```python
from build123d import *

# Parameters (mm, degrees)
PAD001_DEPTH      = 3.3
SKETCH002_W       = 1.5
SKETCH002_H       = 2.9
POCKET_DEPTH      = 5
PAD002_DEPTH      = 0.1
PAD002_DEPTH_BACK = 1


with BuildPart() as part:
    # Sketch001 → Pad001 (new body)
    with BuildSketch(Plane.XY.offset(0.01)):
        Polygon((-7.95, 11), (7.95, 11), (7.95, 0), (-6.95, 0), (-7.95, 1), align=None)
    extrude(amount=PAD001_DEPTH)

    # Sketch002 → Pocket (cut)
    with BuildSketch(Plane.XY.offset(3.31)):
        with Locations((-7.2, 5.5)):
            Rectangle(SKETCH002_W, SKETCH002_H)
        with Locations((7.2, 5.5)):
            Rectangle(SKETCH002_W, SKETCH002_H)
    extrude(amount=-POCKET_DEPTH, mode=Mode.SUBTRACT)

    # Sketch003 → Pad002 (new body, two sides)
    with BuildSketch(Plane(origin=(0, 0, 0.01), x_dir=(1, 0, 0), z_dir=(0, 0, -1))) as pad002_sk:
        Polygon((-7.95, -6.95), (-7.95, -4.05), (-4.8, -4.05), (-4.8, -2.5), (4.8, -2.5), (4.8, -4.05), (7.95, -4.05), (7.95, -6.95), (4.8, -6.95), (4.8, -8.5), (-4.8, -8.5), (-4.8, -6.95), align=None)
    extrude(amount=PAD002_DEPTH)
    extrude(pad002_sk.sketch, amount=-PAD002_DEPTH_BACK)


solid = part.part
```
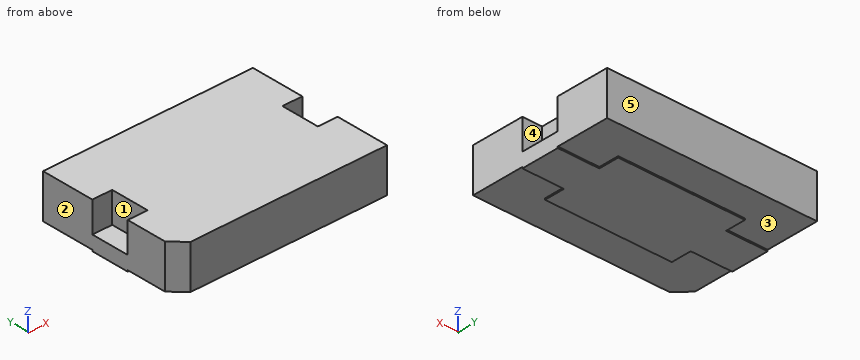
Can you work these out from the model? Positions are in its coordinate system, mm. Face numbers are marked on the shaded views. A direction names the side the tool comes from. Coordinates: 2 decimals unless noted, no trailing zeros. Order: outer loops, then holes, each group sorted by start corner. A loop starts at its lowest first (then second) coordinate and runs counter-clockwise, first axis right, second up. Notation, with made-up numbers: (47.5, 38) - (76.5, 38) arc R29 ccw to (76.5, 77) - close; hole circle Ø8 at (83, 12.5). An arc over 180 degrees is marked (long way). Answer in a Markdown table with one row per item.
1. Suppose I cut it at D-D (y = 1.25). Please give me the cut outline in (x, z), and give its area (3 significant figures).
Reply:
| item | result |
|---|---|
| outline | (-7.95, 0.01) - (7.95, 0.01) - (7.95, 3.31) - (-7.95, 3.31) - close |
| area | 52.5 mm^2 |
2. For the marked faces 1 and 2, which set-ups out of +Z, -Z, +X, -X, +Y, -Y let a thin tool reach every point of the face, with its end or its side?
Reply:
| item | result |
|---|---|
| face 1 | +Z, -X |
| face 2 | +Z, -Z, -X, +Y, -Y |
3. For pin 1 (1.6 mm diameter, centred on x = -7, z = 2, fed in from -Y); pin 2 (1.6 mm diameter, centred on x = 7.5, y = 5, fed in from +Z), each with a flat end and sliding along its axis, tell me the tip position at first contact or that it passes through.
Reply:
| item | result |
|---|---|
| pin 1 | stops at y = 0 |
| pin 2 | stops at z = 1.01 |
4. If I drill on line 1 along Y through (x, z) = (7.5, 2.5); line 2 along Z through (x, y) = (7, 8.5); line 3 along X through (y, z) = (5, 1.85), over which ranges is the centre line in solid material (lowest first)?
Reply:
| item | result |
|---|---|
| line 1 | y = 0 to 4.05, 6.95 to 11 |
| line 2 | z = 0.01 to 3.31 |
| line 3 | x = -6.45 to 6.45 |
5. If we mould it in two halves opening along Y, with no side actions, what happens to the marked faces 3, 4 and 5? For each: pulls with the +Y half, pulls with the -Y half, needs draft (parallel to the pull), parting line crosses it, or undercut.
Reply:
| item | result |
|---|---|
| face 3 | needs draft |
| face 4 | undercut |
| face 5 | pulls with the +Y half |
6. Suppose I cut it at A-A (x = -5). Please give me the cut outline in (y, z).
Reply:
| item | result |
|---|---|
| outline | (0, 0.01) - (4.05, 0.01) - (4.05, -0.09) - (6.95, -0.09) - (6.95, 0.01) - (11, 0.01) - (11, 3.31) - (0, 3.31) - close |
7. Suppose I cut it at B-B (y = 5.75). Please give me the cut outline in (x, z).
Reply:
| item | result |
|---|---|
| outline | (-7.95, -0.09) - (7.95, -0.09) - (7.95, 1.01) - (6.45, 1.01) - (6.45, 3.31) - (-6.45, 3.31) - (-6.45, 1.01) - (-7.95, 1.01) - close |
8. Suppose I cut it at C-C (z = 2.55). Please give me the cut outline in (x, y).
Reply:
| item | result |
|---|---|
| outline | (-7.95, 1) - (-6.95, 0) - (7.95, 0) - (7.95, 4.05) - (6.45, 4.05) - (6.45, 6.95) - (7.95, 6.95) - (7.95, 11) - (-7.95, 11) - (-7.95, 6.95) - (-6.45, 6.95) - (-6.45, 4.05) - (-7.95, 4.05) - close |
